Design review of the part built by this model. Coordinates are the model's own, in mm. A direction names the side the tool comes from. Round coordinates to 2 decimals unless told otherwise and drop trailing zeros. Loops run counter-clockwise (first coordinate to the right, second up) from the corner with the lowest first, then second, coordinate; pieces in that order, holes last. Notation, with made-up numbers: (79, 48.25) - (134, 48.25) arc R15 cw to (134, 75.25) - close; hole circle Ø9 at (76, -33). An arc over 180 degrees is marked (long way). Answer as CSV lines item,"result". Start each with the question number.
(1) Wall thickness on L1, parallel to X at y = -15.5, z = -116.5; L2, parallel to Z at x = -67, y = -3; L3, parallel to Z at x = 64.5, y = -10.75: over which ranges is each line inside the solid? List them lowest first.
(2) Consider section A-A (z = -109). Give the boundary of the cut face in (x, y).
(3) Consider section C-C (y = -17.25). Give the boundary of the cut face in (x, z).
(4) Mouldability with a two-part tool opening along Z and no side actions: class faces 3 (the flat face through (-150, -5, -2)), 4 (the flat face through (-2, -11, -140)), 5 (the flat face through (-2, -11, 140)) as released by +Z, released by -Z, zero draft, split by the parting line, or undercut.
(5) For faces 1 (the flat face through (9, -21, 2)), 2 (the flat face through (-140, -11, 2)), list the 3-axis set-ups (+Z, -Z, +X, -X, +Y, -Y) from which the entire face can be reached by the end or side of a thin tool; tool diameter is ignored.
(6) For P1, Ø1.5, axis at x = -80.5, y = -18, coming from the +Z side; P2, Ø23, axis at x = -143, z = -32.5, coming from the -Y side; P3, Ø12, axis at x = -68.5, y = -10.5, coming from the +Z side, all flat-tipped, find the tip position at first contact; note any pin that passes through.
from build123d import *

# Parameters (mm, degrees)
F0_W     = 300
F0_H     = 302
F1_DEPTH = 21
F2_SIZE  = 20.99999
F3_W     = 21
F3_H     = 302
F4_DEPTH = 10


# Not quite as in the source:
# - a fillet or chamfer is up to 0.001 mm smaller than in the source, because OpenCascade refuses the exact size


with BuildPart() as f1:
    # F0 (on Front) → F1 (new body)
    with BuildSketch(Plane.XZ):
        Rectangle(F0_W, F0_H)
    extrude(amount=F1_DEPTH)

    # F2 (size 21 in the source; OpenCascade refuses exactly that, so slightly less here)
    f2_edges = [f1.edges().sort_by_distance(p)[0] for p in [
        (0, -21, 151),
        (0, -21, -151),
    ]]
    chamfer(f2_edges, length=F2_SIZE)

    # F3 (on face) → F4 (cut)
    with BuildSketch(Plane.XZ.offset(21)):
        with Locations((-139.5, 0)):
            Rectangle(F3_W, F3_H)
    extrude(amount=-F4_DEPTH, mode=Mode.SUBTRACT)


solid = f1.part
Determined:
1,L1,"x = -129 to 150"
1,L2,"z = -148 to 148"
1,L3,"z = -140.25 to 140.25"
2,outline,"(-150, -11) - (-129, -11) - (-129, -21) - (150, -21) - (150, 0) - (-150, 0) - close"
3,outline,"(-129, -133.75) - (150, -133.75) - (150, 133.75) - (-129, 133.75) - close"
4,face 3,"zero draft"
4,face 4,"released by -Z"
4,face 5,"released by +Z"
5,face 1,"+Z, -Z, +X, -X, -Y"
5,face 2,"+Z, -Z, -X, -Y"
6,P1,"stops at z = 133.75"
6,P2,"stops at y = -11"
6,P3,"stops at z = 146.5"
